```python
from build123d import *

# Parameters (mm, degrees)
SKETCH1_R                  = 14
BOSS_EXTRUDE1_DEPTH        = 1.75
M2_5_CLEARANCE_HOLE1_D     = 3.1
M2_5_CLEARANCE_HOLE1_DEPTH = 6
M2_5_CLEARANCE_HOLE1_TIP   = 0.931333959
SKETCH7_R                  = 5
CUT_EXTRUDE1_DEPTH         = 2.3
BOSS_EXTRUDE3_DEPTH        = 3.5
M3_CLEARANCE_HOLE1_D       = 3.6
M3_CLEARANCE_HOLE1_DEPTH   = 6
M3_CLEARANCE_HOLE1_TIP     = 1.081549114


with BuildPart() as part:
    # Sketch1 → Boss-Extrude1 (new, symmetric)
    with BuildSketch(Plane(origin=(0, 0, 0), x_dir=(1, 0, 0), z_dir=(0, 1, 0))):
        with Locations(Location((0, 0, 0), (0, 0, 270))):
            Circle(SKETCH1_R)
    extrude(amount=BOSS_EXTRUDE1_DEPTH, both=True)

    # M2.5 Clearance Hole1
    with Locations(Plane(origin=(0, 1.75, 0), x_dir=(1, 0, 0), z_dir=(0, 1, 0))):
        with Locations((-11, 0), (-7.778174593, 7.778174593), (0, 11), (7.778174593, 7.778174593), (11, 0), (7.778174593, -7.778174593), (0, -11), (-7.778174593, -7.778174593)):
            Hole(M2_5_CLEARANCE_HOLE1_D / 2, depth=M2_5_CLEARANCE_HOLE1_DEPTH)
            with Locations((0, 0, -(M2_5_CLEARANCE_HOLE1_DEPTH + M2_5_CLEARANCE_HOLE1_TIP / 2))):  # 118° drill point
                Cone(0, M2_5_CLEARANCE_HOLE1_D / 2, M2_5_CLEARANCE_HOLE1_TIP, mode=Mode.SUBTRACT)

    # Sketch7 → Cut-Extrude1 (cut)
    with BuildSketch(Plane.XZ.offset(1.75)):
        with Locations(Location((0, 0, 0), (0, 0, 270))):
            Circle(SKETCH7_R)
    extrude(amount=-CUT_EXTRUDE1_DEPTH, mode=Mode.SUBTRACT)

    # Sketch8 → Boss-Extrude3 (add)
    with BuildSketch(Plane(origin=(0, 1.75, 0), x_dir=(1, 0, 0), z_dir=(0, 1, 0))):
        with BuildLine():
            Line((-0.128852443, -2.696923627), (0.057352661, -3.049460718))
            ThreePointArc((0.057352661, -3.049460718), (0.151245078, -3.04624768), (0.244993995, -3.040144395))
            Line((0.244993995, -3.040144395), (0.395362741, -2.670896535))
            ThreePointArc((0.395362741, -2.670896535), (0.470816738, -2.658633408), (0.545893326, -2.644239111))
            Line((0.545893326, -2.644239111), (0.813920864, -2.939393275))
            ThreePointArc((0.813920864, -2.939393275), (0.904064427, -2.912931086), (0.993350224, -2.883705139))
            Line((0.993350224, -2.883705139), (1.047166652, -2.488662694))
            ThreePointArc((1.047166652, -2.488662694), (1.117200406, -2.458020189), (1.18633861, -2.425407327))
            Line((1.18633861, -2.425407327), (1.519347425, -2.644632943))
            ThreePointArc((1.519347425, -2.644632943), (1.600078084, -2.596584319), (1.679290606, -2.546072084))
            Line((1.679290606, -2.546072084), (1.63317323, -2.150057022))
            ThreePointArc((1.63317323, -2.150057022), (1.693386265, -2.102960522), (1.752241875, -2.054178281))
            Line((1.752241875, -2.054178281), (2.1293078, -2.183700596))
            ThreePointArc((2.1293078, -2.183700596), (2.19555295, -2.11708461), (2.259714983, -2.048459957))
            Line((2.259714983, -2.048459957), (2.116561528, -1.676355361))
            ThreePointArc((2.116561528, -1.676355361), (2.163170436, -1.615764111), (2.208045339, -1.553877659))
            Line((2.208045339, -1.553877659), (2.605475935, -1.58555831))
            ThreePointArc((2.605475935, -1.58555831), (2.653073149, -1.504560688), (2.698153157, -1.422135556))
            Line((2.698153157, -1.422135556), (2.466958481, -1.097322127))
            ThreePointArc((2.466958481, -1.097322127), (2.497034654, -1.027043299), (2.525109194, -0.955941189))
            Line((2.525109194, -0.955941189), (2.917932434, -0.887789563))
            ThreePointArc((2.917932434, -0.887789563), (2.943891005, -0.797499685), (2.967056445, -0.706453148))
            Line((2.967056445, -0.706453148), (2.66234736, -0.449340108))
            ThreePointArc((2.66234736, -0.449340108), (2.674001, -0.373789578), (2.683511152, -0.297939418))
            Line((2.683511152, -0.297939418), (3.047044507, -0.134237734))
            ThreePointArc((3.047044507, -0.134237734), (3.049733363, -0.040328844), (3.049528665, 0.053618309))
            Line((3.049528665, 0.053618309), (2.690451163, 0.226875602))
            ThreePointArc((2.690451163, 0.226875602), (2.68295003, 0.302950716), (2.673298235, 0.378782983))
            Line((2.673298235, 0.378782983), (2.984699568, 0.627748746))
            ThreePointArc((2.984699568, 0.627748746), (2.963949757, 0.719376006), (2.940387783, 0.810320731))
            Line((2.940387783, 0.810320731), (2.549504025, 0.888835884))
            ThreePointArc((2.549504025, 0.888835884), (2.523319442, 0.960655502), (2.495112158, 1.031705055))
            Line((2.495112158, 1.031705055), (2.734814978, 1.350291464))
            ThreePointArc((2.734814978, 1.350291464), (2.691930287, 1.433879817), (2.646491522, 1.516107721))
            Line((2.646491522, 1.516107721), (2.248362172, 1.494947338))
            ThreePointArc((2.248362172, 1.494947338), (2.205139413, 1.55799877), (2.160149007, 1.619801305))
            Line((2.160149007, 1.619801305), (2.313091905, 1.987990402))
            ThreePointArc((2.313091905, 1.987990402), (2.250766937, 2.058287685), (2.186306467, 2.126632087))
            Line((2.186306467, 2.126632087), (1.805947455, 2.007125753))
            ThreePointArc((1.805947455, 2.007125753), (1.748402365, 2.057447246), (1.68945575, 2.106119481))
            Line((1.68945575, 2.106119481), (1.74602876, 2.500776593))
            ThreePointArc((1.74602876, 2.500776593), (1.668179623, 2.553365768), (1.588747735, 2.603532338))
            Line((1.588747735, 2.603532338), (1.250058417, 2.393189076))
            ThreePointArc((1.250058417, 2.393189076), (1.181806766, 2.427618744), (1.112607775, 2.460102424))
            Line((1.112607775, 2.460102424), (1.069256207, 2.856429793))
            ThreePointArc((1.069256207, 2.856429793), (0.980774447, 2.888006489), (0.89136214, 2.916843077))
            Line((0.89136214, 2.916843077), (0.615623612, 2.628879527))
            ThreePointArc((0.615623612, 2.628879527), (0.540953902, 2.645254028), (0.465850562, 2.659508085))
            Line((0.465850562, 2.659508085), (0.325298354, 3.032603004))
            ThreePointArc((0.325298354, 3.032603004), (0.231743607, 3.041183141), (0.137968984, 3.046877838))
            Line((0.137968984, 3.046877838), (-0.057493089, 2.699387809))
            ThreePointArc((-0.057493089, 2.699387809), (-0.133889085, 2.696678274), (-0.210177756, 2.691807071))
            Line((-0.210177756, 2.691807071), (-0.439099191, 3.018226615))
            ThreePointArc((-0.439099191, 3.018226615), (-0.531848537, 3.003271072), (-0.624093271, 2.985466059))
            Line((-0.624093271, 2.985466059), (-0.726997287, 2.600283627))
            ThreePointArc((-0.726997287, 2.600283627), (-0.800319329, 2.578660305), (-0.872999832, 2.55496992))
            Line((-0.872999832, 2.55496992), (-1.175906519, 2.814203948))
            ThreePointArc((-1.175906519, 2.814203948), (-1.262022681, 2.776652436), (-1.346941451, 2.736466467))
            Line((-1.346941451, 2.736466467), (-1.350821572, 2.337794062))
            ThreePointArc((-1.350821572, 2.337794062), (-1.416462566, 2.298615626), (-1.480968118, 2.257594612))
            Line((-1.480968118, 2.257594612), (-1.838827315, 2.433354496))
            ThreePointArc((-1.838827315, 2.433354496), (-1.912899299, 2.375566516), (-1.985156345, 2.315524624))
            Line((-1.985156345, 2.315524624), (-1.88976877, 1.928412299))
            ThreePointArc((-1.88976877, 1.928412299), (-1.943604251, 1.874140474), (-1.995881731, 1.818366332))
            Line((-1.995881731, 1.818366332), (-2.386207829, 1.899608433))
            ThreePointArc((-2.386207829, 1.899608433), (-2.443581419, 1.825215014), (-2.498636566, 1.749089852))
            Line((-2.498636566, 1.749089852), (-2.309974846, 1.397861298))
            ThreePointArc((-2.309974846, 1.397861298), (-2.348622132, 1.331906183), (-2.385386754, 1.264883407))
            Line((-2.385386754, 1.264883407), (-2.783654129, 1.246502985))
            ThreePointArc((-2.783654129, 1.246502985), (-2.820724331, 1.160178541), (-2.855118261, 1.072753333))
            Line((-2.855118261, 1.072753333), (-2.585036707, 0.779477531))
            ThreePointArc((-2.585036707, 0.779477531), (-2.606067447, 0.705983328), (-2.625009154, 0.631923206))
            Line((-2.625009154, 0.631923206), (-3.006193202, 0.51507517))
            ThreePointArc((-3.006193202, 0.51507517), (-3.02063076, 0.422243783), (-3.032202376, 0.329011776))
            Line((-3.032202376, 0.329011776), (-2.697671205, 0.112116324))
            ThreePointArc((-2.697671205, 0.112116324), (-2.69976396, 0.035700944), (-2.699692576, -0.040743054))
            Line((-2.699692576, -0.040743054), (-3.0398421, -0.248716711))
            ThreePointArc((-3.0398421, -0.248716711), (-3.030739849, -0.342222105), (-3.018762064, -0.435402801))
            Line((-3.018762064, -0.435402801), (-2.640801099, -0.562289564))
            ThreePointArc((-2.640801099, -0.562289564), (-2.623824375, -0.636824661), (-2.604744383, -0.710849278))
            Line((-2.604744383, -0.710849278), (-2.88248654, -0.996880808))
            ThreePointArc((-2.88248654, -0.996880808), (-2.850416406, -1.085184919), (-2.815641829, -1.172459418))
            Line((-2.815641829, -1.172459418), (-2.417999748, -1.201364731))
            ThreePointArc((-2.417999748, -1.201364731), (-2.383020254, -1.269336231), (-2.346130522, -1.336290227))
            Line((-2.346130522, -1.336290227), (-2.544013749, -1.682407216))
            ThreePointArc((-2.544013749, -1.682407216), (-2.490990819, -1.759961574), (-2.435604463, -1.835846099))
            Line((-2.435604463, -1.835846099), (-2.04326658, -1.764953733))
            ThreePointArc((-2.04326658, -1.764953733), (-1.992482207, -1.822090738), (-1.940100652, -1.877767147))
            Line((-1.940100652, -1.877767147), (-2.045691219, -2.262221792))
            ThreePointArc((-2.045691219, -2.262221792), (-1.975047116, -2.32415337), (-1.902529111, -2.383879817))
            Line((-1.902529111, -2.383879817), (-1.540147459, -2.217644202))
            ThreePointArc((-1.540147459, -2.217644202), (-1.476749174, -2.260356582), (-1.412167122, -2.301257052))
            Line((-1.412167122, -2.301257052), (-1.418830385, -2.699892653))
            ThreePointArc((-1.418830385, -2.699892653), (-1.33500394, -2.742310063), (-1.249910858, -2.782125599))
            Line((-1.249910858, -2.782125599), (-0.940255208, -2.530991929))
            ThreePointArc((-0.940255208, -2.530991929), (-0.86822656, -2.556595909), (-0.795501939, -2.580150512))
            Line((-0.795501939, -2.580150512), (-0.70281922, -2.967919329))
            ThreePointArc((-0.70281922, -2.967919329), (-0.611077556, -2.988157329), (-0.518756109, -3.005560197))
            Line((-0.518756109, -3.005560197), (-0.281283264, -2.685308125))
            ThreePointArc((-0.281283264, -2.685308125), (-0.205150078, -2.692194912), (-0.128852443, -2.696923627))
        make_face()
    extrude(amount=BOSS_EXTRUDE3_DEPTH)

    # M3 Clearance Hole1
    with Locations(Plane(origin=(0, 5.25, 0), x_dir=(1, 0, 0), z_dir=(0, 1, 0))):
        with Locations((0, 0)):
            Hole(M3_CLEARANCE_HOLE1_D / 2, depth=M3_CLEARANCE_HOLE1_DEPTH)
            with Locations((0, 0, -(M3_CLEARANCE_HOLE1_DEPTH + M3_CLEARANCE_HOLE1_TIP / 2))):  # 118° drill point
                Cone(0, M3_CLEARANCE_HOLE1_D / 2, M3_CLEARANCE_HOLE1_TIP, mode=Mode.SUBTRACT)


solid = part.part
```
Design review of the part built by this model. Coordinates are the model's own, in mm. A direction names the side the tool comes from. Round coordinates to 2 decimals unless told otherwise and drop trailing zeros. Write each loop counter-clockwise with the first axis right and the second up, starting at its lowest first coordinate (ties: lowest second). Pieces come first, ordered by that corner, then holes. Notation, with made-up numbers: (83.5, -5.5) -> (128.5, -5.5) arc R26 ccw to (128.5, 28.5) -> close; hole circle Ø1 at (4.25, -11). An arc over 180 degrees is marked (long way). Answer in a Markdown table with one row per item.
Q1. To check wall thickness, follow L1, parallel to Z at x = -8.5, y = -0.75; L2, parallel to Z at x = 8, y = 0.5. State the ranges of each line that lie inside material, in increasing order. Write a range as [from, to].
The answers:
| item | result |
|---|---|
| L1 | [-11.12, -9.15], [-6.41, 6.41], [9.15, 11.12] |
| L2 | [-11.49, -9.31], [-6.24, 6.24], [9.31, 11.49] |
Q2. Take a section at D-D, the plane z = -11. State the section outline as (x, y) points, then the cut area to 3 significant figures.
The answers:
| item | result |
|---|---|
| outline | (-8.66, -1.75) -> (-1.55, -1.75) -> (-1.55, 1.75) -> (-8.66, 1.75) -> close; (1.55, -1.75) -> (8.66, -1.75) -> (8.66, 1.75) -> (1.55, 1.75) -> close |
| area | 49.8 mm² |
Q3. Take a section at B-B, the plane z = 10. State the section outline as (x, y) points.
The answers:
| item | result |
|---|---|
| outline | (-9.8, -1.75) -> (-1.18, -1.75) -> (-1.18, 1.75) -> (-9.8, 1.75) -> close; (1.18, -1.75) -> (9.8, -1.75) -> (9.8, 1.75) -> (1.18, 1.75) -> close |
Q4. Clearance check with flat-ended pins moving along their axes: pin 1 Ø4 at (x, y) = (4.5, 0.5) entering from -Z (3 decimals); pin 2 Ø2.5 at (x, z) = (-11, 0) entering from +Y; pin 3 Ø3.5 at (x, z) = (7.78, 7.78) entering from +Y; pin 4 Ø2 at (y, z) = (2.5, -6.5) entering from +X. State where each tip first meets the part, or that it passes through.
The answers:
| item | result |
|---|---|
| pin 1 | z = -13.775 |
| pin 2 | through |
| pin 3 | y = 1.75 |
| pin 4 | x = 12.72 |
Q5. Draft analysis for pull direction Z (two halves, no side actions). For faces 3 (the face through (-9.77, -0.02, 0.94)), 4 (the face through (-13.67, 0.02, -3.03)), 5 (the face through (-6, -1.75, 0)), state which applies: +Z half, -Z half, draft (parallel to the pull), parting line (faces both ways), or undercut.
The answers:
| item | result |
|---|---|
| face 3 | undercut |
| face 4 | parting line |
| face 5 | draft |
Q6. Take a section at C-C, the plane y = -1. Count the separate pieces of the cut face and the enclosed holes in it, then the cut area to 3 significant figures.
The answers:
| item | result |
|---|---|
| separate pieces | 1 |
| enclosed holes | 9 |
| area | 477 mm² |
Q7. For faces 1 (the face through (0, 0.55, -2)), 2 (the face through (0.336, -0.024, 12.513)), list the 3-axis set-ups (+Z, -Z, +X, -X, +Y, -Y) from which the entire face can be reached by the end or side of a thin tool; tool diameter is ignored.
The answers:
| item | result |
|---|---|
| face 1 | -Y |
| face 2 | +Y, -Y |
Q8. Take a section at A-A, the plane x = -9. State the section outline as (y, z) points.
The answers:
| item | result |
|---|---|
| outline | (-1.75, -10.72) -> (1.75, -10.72) -> (1.75, -8.73) -> (-1.75, -8.73) -> close; (-1.75, -6.82) -> (1.75, -6.82) -> (1.75, 6.82) -> (-1.75, 6.82) -> close; (-1.75, 8.73) -> (1.75, 8.73) -> (1.75, 10.72) -> (-1.75, 10.72) -> close |
